Design review of the part built by this model. Coordinates are the model's own, in mm. A direction names the side the tool comes from. Give positions to 0.01 mm unless a question says otherwise; leave off trailing zeros. Write each loop counter-clockwise with the first axis right and the second up, starting at its lowest first coordinate (ties: lowest second). Pieces come first, ordered by that corner, then holes. Notation, with made-up numbers: M 61,47 L 82,47 A24 cw 82,74 Z; hole C 23.25,-14.75 d5. An arc over 180 degrees is marked long. Use a Markdown table: item, result. Add a question column.
```python
from build123d import *

# Parameters (mm, degrees)
FILLET1_R          = 6.35
SKETCH2_R          = 34.925
CUT_EXTRUDE1_DEPTH = 3.175
FILLET2_R          = 1.27


with BuildPart() as part:
    # Sketch1 → Revolve1 (revolve)
    with BuildSketch(Plane(origin=(0, 0, 0), x_dir=(0, 0, -1), z_dir=(1, 0, 0))):
        Polygon((-76.2, 25.087112537), (-53.975, 9.525), (-50.8, 9.525), (76.2, 31.91852655), (76.2, 38.1), (-63.5, 38.1), (-63.5, 56.388), (-76.2, 56.388), align=None)
    revolve(axis=Axis((0, 0, 76.2), (0, 0, -1)))

    # Fillet1
    fillet1_edges = [part.edges().sort_by_distance(p)[0] for p in [
        (0, -38.1, 63.5),
    ]]
    fillet(fillet1_edges, radius=FILLET1_R)

    # Sketch2 → Cut-Extrude1 (cut)
    with BuildSketch(Plane.XY.offset(76.2)):
        Circle(SKETCH2_R)
    extrude(amount=-CUT_EXTRUDE1_DEPTH, mode=Mode.SUBTRACT)

    # Fillet2
    fillet2_edges = [part.edges().sort_by_distance(p)[0] for p in [
        (-34.925, 0, 73.025),
    ]]
    fillet(fillet2_edges, radius=FILLET2_R)


solid = part.part
```
(1) Wall thickness on L1, parallel to X at y = 0, z = 51.7 (3 decimals); L2, parallel to Z at x = -33.5, y = -39.5; L3, parallel to X at y = 0, z = -26: over which ranges is each line inside the solid? List them lowest first.
(2) For pin 1 (10 mm diameter, centred on x = 38.5, y = 32.5, fed in from -Z); pin 2 (10 mm diameter, centred on y = -8, z = -5.5, fed in from -X); pin 3 (1.5 mm diameter, centred on x = -9, z = -13, fed in from -Y); pin 4 (17 mm diameter, centred on x = 0, y = 0, fed in from -Z), all flat-tipped, find the tip position at first contact; note any pin that passes through.
(3) Add section A-A on y = 0. Give the boundary of the cut face in (x, z) (3 decimals), then the cut area to 3 significant figures.
(4) Add section C-C on z = 4.5. Give the boundary of the cut face in (x, y), then the cut area to 3 significant figures.
(5) Add section D-D on z = -48. Give the boundary of the cut face in (x, y).
(6) Machinability: for faces 1 (the cylindrical face through (-23.183, -30.235, -8.592)), 2 (the flat face through (7, -22, 73.025)), 3 (the flat face through (-31, 9, -76.2)), which of the approach directions +Z, -Z, +X, -X, +Y, -Y give a long, thin tool a straight path to every point of the face, cutting with its end or side? Answer none if there is none.
(7) The part is to be moulded in two halves that separate along Y. For faces 4 (the cylindrical face through (-5.796, -7.559, 52.365)), 5 (the flat face through (17, -42, 63.5)), 6 (the cylindrical face through (-34.31, -44.75, 69.94)), 7 (the conical face through (-9.93, -2.21, 54.9)), say which applies: released by +Y, released by -Y, zero draft, split by the parting line, or undercut.
From the geometry:
| question | item | result |
|---|---|---|
| 1 | L1 | x = -38.1 to -9.525, 9.525 to 38.1 |
| 1 | L2 | z = 63.5 to 76.2 |
| 1 | L3 | x = -38.1 to -23.07, 23.07 to 38.1 |
| 2 | pin 1 | stops at z = 63.5 |
| 2 | pin 2 | stops at x = -37.98 |
| 2 | pin 3 | stops at y = -37.2 |
| 2 | pin 4 | passes through |
| 3 | outline | M -56.388,63.5 L -44.45,63.5 A6.35 cw -38.1,57.15 L -38.1,-76.2 L -31.919,-76.2 L -9.525,50.8 L -9.525,53.975 L -22.864,73.025 L -33.655,73.025 A1.27 cw -34.925,74.295 L -34.925,76.2 L -56.388,76.2 Z; M 9.525,50.8 L 31.919,-76.2 L 38.1,-76.2 L 38.1,57.15 A6.35 cw 44.45,63.5 L 56.388,63.5 L 56.388,76.2 L 34.925,76.2 L 34.925,74.295 A1.27 cw 33.655,73.025 L 22.864,73.025 L 9.525,53.975 Z |
| 3 | area | 5,930 mm^2 |
| 4 | outline | C 0,0 d76.2; hole C 0,0 d35.38 |
| 4 | area | 3,580 mm^2 |
| 5 | outline | C 0,0 d76.2; hole C 0,0 d53.89 |
| 6 | face 1 | -Z |
| 6 | face 2 | +Z |
| 6 | face 3 | -Z, +X, -X, +Y, -Y |
| 7 | face 4 | undercut |
| 7 | face 5 | zero draft |
| 7 | face 6 | split by the parting line |
| 7 | face 7 | undercut |
